from build123d import *

# Parameters (mm, degrees)
F0_R     = 9
F0_R_2   = 8.5
F0_W     = 2
F0_H     = 20
F1_DEPTH = 20
F2_DEPTH = 0.5
F3_DEPTH = 16


with BuildPart() as f1:
    # F0 (on Front) → F1 (new body, symmetric)
    with BuildSketch(Plane.XZ):
        with BuildLine():
            Line((20, -20), (20, 0))
            ThreePointArc((20, 0), (0, 20), (-20, 0))
            Line((-20, 0), (-20, -20))
            Line((-20, -20), (20, -20))
        make_face()
        Circle(F0_R, mode=Mode.SUBTRACT)
        with BuildLine():
            ThreePointArc((-20, 0), (0, 20), (20, 0))
            Line((20, 0), (22, 0))
            ThreePointArc((22, 0), (0, 22), (-22, 0))
            Line((-22, 0), (-22, -20))
            Line((-22, -20), (-20, -20))
            Line((-20, -20), (-20, 0))
        make_face()
        with Locations((21, -10)):
            Rectangle(F0_W, F0_H)
        Circle(F0_R)
        Circle(F0_R_2, mode=Mode.SUBTRACT)
    extrude(amount=F1_DEPTH, both=True)

    # F0 (on Front) → F2 (cut, symmetric)
    with BuildSketch(Plane.XZ):
        Circle(F0_R)
        Circle(F0_R_2, mode=Mode.SUBTRACT)
    extrude(amount=F2_DEPTH, both=True, mode=Mode.SUBTRACT)

    # F0 (on Front) → F3 (cut, symmetric)
    with BuildSketch(Plane.XZ):
        with BuildLine():
            ThreePointArc((-20, 0), (0, 20), (20, 0))
            Line((20, 0), (22, 0))
            ThreePointArc((22, 0), (0, 22), (-22, 0))
            Line((-22, 0), (-22, -20))
            Line((-22, -20), (-20, -20))
            Line((-20, -20), (-20, 0))
        make_face()
        with Locations((21, -10)):
            Rectangle(F0_W, F0_H)
    extrude(amount=F3_DEPTH, both=True, mode=Mode.SUBTRACT)


solid = f1.part
Can you work these out from the model? Positions are in its coordinate system, mm. A direction names the side the tool comes from. Give positions to 0.01 mm unless a question says otherwise; leave off trailing zeros. Order: outer loops, then holes, each group sorted by start corner. A loop starts at its lowest first (then second) coordinate and runs counter-clockwise, first axis right, second up. Notation, with made-up numbers: M 40,82.25 L 99,82.25 A32 cw 99,112.25 Z; hole C -15.5,29 d8. An arc over 180 degrees is marked long. One line per question, with ' | ' between items.
Item 1: Suppose I cut it at D-D, the plane z = -11. Write out the boundary of the cut face in (x, y).
Answer block:
outline: M -22,-20 L 22,-20 L 22,-16 L 20,-16 L 20,16 L 22,16 L 22,20 L -22,20 L -22,16 L -20,16 L -20,-16 L -22,-16 Z
Item 2: We'd pull the mould along Z, two halves only. Please class faces 1 (the face through (4.57, -10.114, 7.167)), 2 (the face through (0, 0, -20)), 3 (the face through (-1.172, -0.007, 8.923)), 4 (the face through (20, 0, -10)): released by +Z, released by -Z, zero draft, split by the parting line, or undercut.
Answer block:
face 1: undercut | face 2: released by -Z | face 3: undercut | face 4: zero draft
Item 3: I'm going to push flat-ended pins straight in: pin 1 Ø10 at (y, z) = (-15, 7) entering from -X; pin 2 Ø2 at (y, z) = (16, 2.5) entering from +X; pin 3 Ø1.5 at (x, y) = (2, -2.5) entering from +Z; pin 4 Ø14.5 at (x, z) = (0, 0) entering from -Y. Where does each tip first touch, or does it pass through?
Answer block:
pin 1: stops at x = -21.9 | pin 2: stops at x = 21.95 | pin 3: stops at z = 19.96 | pin 4: passes through
Item 4: Suppose I cut it at C-C, the plane y = 9. Write out the boundary of the cut face in (x, z), then the cut area to 3 significant figures.
Answer block:
outline: M -20,-20 L 20,-20 L 20,0 A20 ccw -20,0 Z; hole C 0,0 d17 | area: 1,200 mm2
Item 5: Suppose I cut it at B-B, the plane z = 6.5. Write out the boundary of the cut face in (x, y), then the cut area to 3 significant figures.
Answer block:
outline: M -21.02,-20 L -5.48,-20 L -5.48,-0.5 L -6.22,-0.5 L -6.22,0.5 L -5.48,0.5 L -5.48,20 L -21.02,20 L -21.02,16 L -18.91,16 L -18.91,-16 L -21.02,-16 Z; M 5.48,-20 L 21.02,-20 L 21.02,-16 L 18.91,-16 L 18.91,16 L 21.02,16 L 21.02,20 L 5.48,20 L 5.48,0.5 L 6.22,0.5 L 6.22,-0.5 L 5.48,-0.5 Z | area: 1,110 mm2
Item 6: Please list where these lines run through material, in increasing order: L1, parallel to Z at x = 0, y = 0.3; L2, parallel to X at y = -5, z = -11; L3, parallel to X at y = 9, z = 1.
Answer block:
L1: z = -20 to -9, 9 to 20 | L2: x = -20 to 20 | L3: x = -19.97 to -8.44, 8.44 to 19.97
Item 7: Suppose I cut it at A-A, the plane x = 0. Write out the boundary of the cut face in (y, z), then the cut area to 3 significant figures.
Answer block:
outline: M -20,-20 L 20,-20 L 20,-8.5 L 0.5,-8.5 L 0.5,-9 L -0.5,-9 L -0.5,-8.5 L -20,-8.5 Z; M -20,8.5 L -0.5,8.5 L -0.5,9 L 0.5,9 L 0.5,8.5 L 20,8.5 L 20,22 L 16,22 L 16,20 L -16,20 L -16,22 L -20,22 Z | area: 935 mm2
Item 8: For faces 5 (the face through (0, 0, 20)), 6 (the face through (-20, 0, -10)), 7 (the face through (8, 0.5, -3.3)), which set-ups out of +Z, -Z, +X, -X, +Y, -Y let a thin tool reach every point of the face, with its end or its side?
Answer block:
face 5: +Z | face 6: +Z, -Z, -X | face 7: none
